Part model, mm, in its own coordinate system. A direction names the side the tool comes from. Round coordinates to 2 decimals unless told otherwise and drop trailing zeros. Write each loop counter-clockwise with the first axis right and the second up, starting at its lowest first coordinate (ties: lowest second). Pieces come first, ordered by that corner, then holes.
from build123d import *

# Parameters (mm, degrees)
SKETCH_1_W               = 31.418685122
SKETCH_1_H               = 20
EXTRUDE_1_DEPTH          = 20
CUT_EXTRUDE_1_DEPTH      = 40
SKETCH_5_OUTSIDE_W       = 44.348
SKETCH_5_OUTSIDE_H       = 32.93
SKETCH_5_OUTSIDE_R       = 9.75
CUT_EXTRUDE_2_DEPTH      = 45.122368972
CUT_EXTRUDE_3_DEPTH      = 1
SKETCH_6_R               = 9.75
CUT_EXTRUDE_4_DEPTH      = 18.50523648
SKETCH_7_W               = 25
SKETCH_7_H               = 22
EXTRUDE_2_DEPTH          = 3
CUT_EXTRUDE_5_DEPTH      = 25.793531221
CUT_EXTRUDE_5_DEPTH_BACK = 25.793531221
SKETCH_8_W               = 31.739015686
SKETCH_8_H               = 6.741185812
SKETCH_9_W               = 2
SKETCH_9_H               = 2
EXTRUDE_3_DEPTH          = 13
SKETCH_10_W              = 3
SKETCH_10_H              = 25
EXTRUDE_4_DEPTH          = 2
SKETCH_11_R              = 0.75
CUT_EXTRUDE_6_DEPTH      = 4
SKETCH_13_R              = 0.9
CUT_EXTRUDE_7_DEPTH      = 27.529322999


with BuildPart() as part:
    # 草图1 → 凸台-拉伸1 (new, symmetric)
    with BuildSketch(Plane(origin=(0, 0, 0), x_dir=(0, 0, -1), z_dir=(1, 0, 0))):
        Rectangle(SKETCH_1_W, SKETCH_1_H)
    extrude(amount=EXTRUDE_1_DEPTH, both=True)

    # 草图2 → 切除-拉伸1 (cut)
    with BuildSketch(Plane(origin=(0, 0, -15.709342561), x_dir=(-1, 0, 0), z_dir=(0, 0, -1))):
        Polygon((-20, 10), (0, 10), (-20, -10), align=None)
    extrude(amount=-CUT_EXTRUDE_1_DEPTH, mode=Mode.SUBTRACT)

    # 草图5 outside → 切除-拉伸2 (cut, through all)
    with BuildSketch(Plane.ZY.offset(20)):
        Rectangle(SKETCH_5_OUTSIDE_W, SKETCH_5_OUTSIDE_H)
        Circle(SKETCH_5_OUTSIDE_R, mode=Mode.SUBTRACT)
    extrude(amount=-CUT_EXTRUDE_2_DEPTH, mode=Mode.SUBTRACT)

    # 草图3 → 切除-拉伸3 (cut)
    with BuildSketch(Plane(origin=(5, 5, 0), x_dir=(0, 0, -1), z_dir=(0.7071067811865477, 0.7071067811865475, 0))):
        Polygon((-7, -12.765541439), (-5, -12.765541439), (-5, -21.213203436), (5, -21.213203436), (5, -12.765541439), (7, -12.765541439), (7, 1.234458561), (-7, 1.234458561), align=None)
    extrude(amount=-CUT_EXTRUDE_3_DEPTH, mode=Mode.SUBTRACT)

    # 草图6 → 切除-拉伸4 (cut)
    with BuildSketch(Plane.ZY.offset(20)):
        Circle(SKETCH_6_R)
    extrude(amount=-CUT_EXTRUDE_4_DEPTH, mode=Mode.SUBTRACT)

    # 草图7 → 凸台-拉伸2 (add)
    with BuildSketch(Plane.ZY.offset(1.49476352)):
        Rectangle(SKETCH_7_W, SKETCH_7_H)
    extrude(amount=EXTRUDE_2_DEPTH)

    # 草图8 → 切除-拉伸5 (cut, two sides: drawn at the far end of the back side and taken through both)
    with BuildSketch(Plane.XY.offset(-CUT_EXTRUDE_5_DEPTH_BACK)):
        with Locations((7.322399495, -9.529036855)):
            Rectangle(SKETCH_8_W, SKETCH_8_H)
    extrude(amount=CUT_EXTRUDE_5_DEPTH + CUT_EXTRUDE_5_DEPTH_BACK, mode=Mode.SUBTRACT)

    # 草图9 → 凸台-拉伸3 (add)
    with BuildSketch(Plane.ZY.offset(4.49476352)):
        with Locations((-9.75, 0)):
            Rectangle(SKETCH_9_W, SKETCH_9_H)
        with Locations((9.75, 0)):
            Rectangle(SKETCH_9_W, SKETCH_9_H)
    extrude(amount=-EXTRUDE_3_DEPTH)

    # 草图10 → 凸台-拉伸4 (add)
    with BuildSketch(Plane.XZ.offset(6.158443949)):
        with Locations((-2.99476352, 0)):
            Rectangle(SKETCH_10_W, SKETCH_10_H)
    extrude(amount=EXTRUDE_4_DEPTH)

    # 草图11 → 切除-拉伸6 (cut)
    with BuildSketch(Plane.ZY.offset(4.49476352)):
        with Locations((0, 3.720778025)):
            Circle(SKETCH_11_R)
        with Locations((2.3, 1.420778025)):
            Circle(SKETCH_11_R)
        with Locations((0, -0.879221975)):
            Circle(SKETCH_11_R)
        with Locations((-2.3, 1.420778025)):
            Circle(SKETCH_11_R)
    extrude(amount=-CUT_EXTRUDE_6_DEPTH, mode=Mode.SUBTRACT)

    # 草图13 → 切除-拉伸7 (cut, through all)
    with BuildSketch(Plane.ZY.offset(4.49476352)):
        with Locations((-9.5, 8.700986726)):
            Circle(SKETCH_13_R)
        with Locations((9.5, 8.700986726)):
            Circle(SKETCH_13_R)
    extrude(amount=-CUT_EXTRUDE_7_DEPTH, mode=Mode.SUBTRACT)


solid = part.part
Q1. Wall check: line 1 (Y direction, x = -3.35, z = 0); line 2 (Y direction, x = -3.65, z = 9.5); line 3 (X direction, y = 5.75, z = 9). Give the ranges that are in metal, low to high.
Q2. Saw through at C-C, the plane x = 1.75. Write the cut outline in (y, z), and give its area (3 significant figures).
Q3. Tool access for faces 1 (the flat face through (14.5, -5.2, -5)), 2 (the flat face through (3, -1, -10)), 3 (the cylindrical face through (-2.523, 4.464, -0.098)): list every direction of +Z, -Z, +X, -X, +Y, -Y with a clear straight run to the whole face (end or side of a thin tool).
Q4. Saw through at D-D, the plane y = 5.5. Write the cut outline in (x, z), and give its area (3 significant figures).
Q5. Two-plate mould, pull along Z, no slides. Class faces 4 (the flat face through (3, 1, 10)), 5 (the flat face through (-0.495, 1, -2)), 6 (the flat face through (-3, 2, 12.5)): released by +Z, released by -Z, zero draft, split by the parting line, or undercut.
Q6. Saw through at B-B, the plane z = 0. Write the cut outline in (x, y).
Q7. Drop flat-ended pins along their axis: P1, Ø10, axis at x = 5.5, y = 0.5, coming from the +Z side; P2, Ø0.6, axis at x = 15, y = -5, coming from the -Z side; P3, Ø7.5, axis at x = 9.5, z = -1, coming from the -Y side. Give the stop position or say it passes through.
Q8. Saw through at A-A, the plane x = -2.25. Write the cut outline in (y, z).
Computed:
1. line 1: y = -8.16 to -1.63, -0.13 to 2.97, 4.47 to 11
1. line 2: y = -8.16 to 7.8, 9.6 to 11
1. line 3: x = -4.49 to -1.49
2. outline: (-6.16, -7.56) arc R9.75 ccw to (-1, -9.7) - (-1, -10.75) - (1, -10.75) - (1, -9.7) arc R9.75 ccw to (8.25, -5.2) - (8.25, 5.2) arc R9.75 ccw to (1, 9.7) - (1, 10.75) - (-1, 10.75) - (-1, 9.7) arc R9.75 ccw to (-6.16, 7.56) - close
2. area: 254 mm2
3. face 1: +X, +Y
3. face 2: -Z, +X, -Y
3. face 3: -X
4. outline: (-4.49, -12.5) - (-1.49, -12.5) - (-1.49, -8.05) - (4.5, -8.05) - (4.5, -7) - (3.75, -7) - (3.75, 7) - (4.5, 7) - (4.5, 8.05) - (-1.49, 8.05) - (-1.49, 12.5) - (-4.49, 12.5) - close
4. area: 161 mm2
5. face 4: zero draft
5. face 5: undercut
5. face 6: released by +Z
6. outline: (-4.49, -8.16) - (-1.49, -8.16) - (-1.49, -6.16) - (14.74, -6.16) - (3.42, 5.17) - (4.13, 5.87) - (0.25, 9.75) - (-1.49, 9.75) - (-1.49, 11) - (-4.49, 11) - (-4.49, 4.47) - (-0.49, 4.47) - (-0.49, 2.97) - (-4.49, 2.97) - (-4.49, -0.13) - (-0.49, -0.13) - (-0.49, -1.63) - (-4.49, -1.63) - close
7. P1: stops at z = 10.75
7. P2: stops at z = -8.49
7. P3: stops at y = -6.16
8. outline: (-8.16, -12.5) - (11, -12.5) - (11, 12.5) - (-8.16, 12.5) - close; hole circle Ø1.5 at (-0.88, 0); hole circle Ø1.5 at (1.42, -2.3); hole circle Ø1.5 at (1.42, 2.3); hole circle Ø1.5 at (3.72, 0); hole circle Ø1.8 at (8.7, -9.5); hole circle Ø1.8 at (8.7, 9.5)
